Read the model definition and answer for the solid it produces. Units are mm, in the model's axes. Round coordinates to 2 decimals unless told otherwise and drop trailing zeros. Order: outer loops, then holes, each group sorted by start corner. A loop starts at its lowest first (then second) coordinate and runs counter-clockwise, first axis right, second up. Notation, with made-up numbers: (2.25, -34.75) - (14.25, -34.75) arc R24 cw to (14.25, -15.75) - close; hole circle Ø5 at (47.5, 58). An arc over 180 degrees is marked (long way). Put each result on its own line as item: value. Start each with the question number.
Q1. Find the intervals of material crossed by line 1 along Y through (x, z) = (-1, -16); line 2 along Z through (x, y) = (32, -6); line 3 along X through (y, z) = (-4.75, 69), in increasing order. Write a range as from..to.
Q2. Section B-B on x = -33 is taken. Give the vertices of the cut face in (y, z), then the cut area to 3 significant figures.
Q3. Section A-A on z = 12 is taken. Give the vertices of the cut face in (x, y).
Q4. For a pull along Z with two mould halves and no side action, classify faces 1 (the face through (-38.5, -5, 1)), 2 (the face through (-1, -10.8, 1)), 3 (the face through (35.794, -5.324, -73.684)), 4 (the face through (-35.794, -5.324, 73.684)) as pulls with the +Z half, pulls with the -Z half, needs draft (parallel to the pull), parting line crosses it, or undercut.
Q5. This flat-tipped pin is pushed along its axis until it touches: pin 1 Ø1.5 at (x, z) = (19, -8.5) entering from -Y. Where does it stop, or does it pass through?
from build123d import *

# Parameters (mm, degrees)
F0_W     = 52.1
F0_H     = 4
F0_R     = 6.1
F1_DEPTH = 10.8
F2_DEPTH = 11


with BuildPart() as f1:
    # F0 (on Front) → F1 (new body)
    with BuildSketch(Plane.XZ):
        with BuildLine():
            Line((-29.5, -76.25), (29.5, -76.25))
            ThreePointArc((29.5, -76.25), (35.863961, -73.613961), (38.5, -67.25))
            Line((38.5, -67.25), (38.5, 67.25))
            ThreePointArc((38.5, 67.25), (35.863961, 73.613961), (29.5, 76.25))
            Line((29.5, 76.25), (-29.5, 76.25))
            ThreePointArc((-29.5, 76.25), (-35.863961, 73.613961), (-38.5, 67.25))
            Line((-38.5, 67.25), (-38.5, -67.25))
            ThreePointArc((-38.5, -67.25), (-35.863961, -73.613961), (-29.5, -76.25))
        make_face()
        with Locations((0, -62.75)):
            Rectangle(F0_W, F0_H, mode=Mode.SUBTRACT)
        with BuildLine():
            Line((-13.786121, 58.25), (-13.786121, 56.25))
            ThreePointArc((-13.786121, 56.25), (-14.371908, 54.835786), (-15.786121, 54.25))
            ThreePointArc((-15.786121, 54.25), (-17.200335, 54.835786), (-17.786121, 56.25))
            Line((-17.786121, 56.25), (-17.786121, 58.25))
            ThreePointArc((-17.786121, 58.25), (-17.200335, 59.664214), (-15.786121, 60.25))
            ThreePointArc((-15.786121, 60.25), (-14.371908, 59.664214), (-13.786121, 58.25))
        make_face(mode=Mode.SUBTRACT)
        with BuildLine():
            Line((3.05, 42.301566), (3.05, 26.101566))
            ThreePointArc((3.05, 26.101566), (2.156676, 23.94489), (0, 23.051566))
            ThreePointArc((0, 23.051566), (-2.156676, 23.94489), (-3.05, 26.101566))
            Line((-3.05, 26.101566), (-3.05, 42.301566))
            ThreePointArc((-3.05, 42.301566), (-2.156676, 44.458242), (0, 45.351566))
            ThreePointArc((0, 45.351566), (2.156676, 44.458242), (3.05, 42.301566))
        make_face(mode=Mode.SUBTRACT)
        with Locations((0, 57.25)):
            Circle(F0_R, mode=Mode.SUBTRACT)
        with BuildLine():
            Line((15.011477, 58.05), (15.011477, 56.45))
            ThreePointArc((15.011477, 56.45), (14.425691, 55.035786), (13.011477, 54.45))
            ThreePointArc((13.011477, 54.45), (11.597264, 55.035786), (11.011477, 56.45))
            Line((11.011477, 56.45), (11.011477, 58.05))
            ThreePointArc((11.011477, 58.05), (11.597264, 59.464214), (13.011477, 60.05))
            ThreePointArc((13.011477, 60.05), (14.425691, 59.464214), (15.011477, 58.05))
        make_face(mode=Mode.SUBTRACT)
    extrude(amount=F1_DEPTH)

    # F0 (on Front) → F2 (join)
    with BuildSketch(Plane.XZ):
        with Locations((0, 57.25)):
            Circle(F0_R)
        with BuildLine():
            ThreePointArc((-15.786121, 54.25), (-14.371908, 54.835786), (-13.786121, 56.25))
            Line((-13.786121, 56.25), (-13.786121, 58.25))
            ThreePointArc((-13.786121, 58.25), (-14.371908, 59.664214), (-15.786121, 60.25))
            ThreePointArc((-15.786121, 60.25), (-17.200335, 59.664214), (-17.786121, 58.25))
            Line((-17.786121, 58.25), (-17.786121, 56.25))
            ThreePointArc((-17.786121, 56.25), (-17.200335, 54.835786), (-15.786121, 54.25))
        make_face()
        with BuildLine():
            ThreePointArc((13.011477, 54.45), (14.425691, 55.035786), (15.011477, 56.45))
            Line((15.011477, 56.45), (15.011477, 58.05))
            ThreePointArc((15.011477, 58.05), (14.425691, 59.464214), (13.011477, 60.05))
            ThreePointArc((13.011477, 60.05), (11.597264, 59.464214), (11.011477, 58.05))
            Line((11.011477, 58.05), (11.011477, 56.45))
            ThreePointArc((11.011477, 56.45), (11.597264, 55.035786), (13.011477, 54.45))
        make_face()
        with BuildLine():
            ThreePointArc((0, 23.051566), (2.156676, 23.94489), (3.05, 26.101566))
            Line((3.05, 26.101566), (3.05, 42.301566))
            ThreePointArc((3.05, 42.301566), (2.156676, 44.458242), (0, 45.351566))
            ThreePointArc((0, 45.351566), (-2.156676, 44.458242), (-3.05, 42.301566))
            Line((-3.05, 42.301566), (-3.05, 26.101566))
            ThreePointArc((-3.05, 26.101566), (-2.156676, 23.94489), (0, 23.051566))
        make_face()
        with Locations((0, -62.75)):
            Rectangle(F0_W, F0_H)
    extrude(amount=F2_DEPTH)


solid = f1.part
Findings:
1. line 1: -10.8..0
1. line 2: -75.9..75.9
1. line 3: -38.33..38.33
2. outline: (-10.8, -75.54) - (0, -75.54) - (0, 75.54) - (-10.8, 75.54) - close
2. area: 1,630 mm2
3. outline: (-38.5, -10.8) - (38.5, -10.8) - (38.5, 0) - (-38.5, 0) - close
4. face 1: needs draft
4. face 2: undercut
4. face 3: pulls with the -Z half
4. face 4: pulls with the +Z half
5. pin 1: y = -10.8
